Geometry check sheet. Reference: the model listing, model coordinates, mm. Coordinates: 2 decimals unless noted, no trailing zeros. Write each loop counter-clockwise with the first axis right and the second up, starting at its lowest first coordinate (ties: lowest second). Pieces come first, ordered by that corner, then holes. Notation, with made-up numbers: (-1, 64) -> (43, 64) arc R38 ccw to (43, 102) -> close; hole circle Ø7 at (-21, 10). An arc over 180 degrees is marked (long way). Use a Markdown table: item, result.
```python
from build123d import *

# Parameters (mm, degrees)
SKETCH2_R           = 1.5
SKETCH2_R_2         = 1
SKETCH2_W           = 3
SKETCH2_H           = 4.5
BOSS_EXTRUDE1_DEPTH = 3


with BuildPart() as part:
    # Sketch2 → Boss-Extrude1 (new body)
    with BuildSketch(Plane(origin=(0, 0, 0), x_dir=(1, 0, 0), z_dir=(0, 1, 0))):
        with BuildLine():
            Line((-90, 8.416796225), (-160, 8.416796225))
            Line((-160, 8.416796225), (-160, 40.416796225))
            Line((-160, 40.416796225), (-136, 40.416796225))
            Line((-136, 40.416796225), (-136, 43.416796225))
            Line((-136, 43.416796225), (-126, 43.416796225))
            Line((-126, 43.416796225), (-126, 40.416796225))
            Line((-126, 40.416796225), (-102, 40.416796225))
            Line((-102, 40.416796225), (-102, 43.416796225))
            Line((-102, 43.416796225), (-92, 43.416796225))
            Line((-92, 43.416796225), (-92, 40.416796225))
            Line((-92, 40.416796225), (-77, 40.416796225))
            Line((-77, 40.416796225), (-77, 37.316796225))
            Line((-77, 37.316796225), (-78.3, 37.316796225))
            Line((-78.3, 37.316796225), (-78.3, 34.816796225))
            Line((-78.3, 34.816796225), (-77, 34.816796225))
            Line((-77, 34.816796225), (-77, 31.016796225))
            Line((-77, 31.016796225), (-74, 31.016796225))
            Line((-74, 31.016796225), (-74, 34.816796225))
            Line((-74, 34.816796225), (-72.7, 34.816796225))
            Line((-72.7, 34.816796225), (-72.7, 37.316796225))
            Line((-72.7, 37.316796225), (-74, 37.316796225))
            Line((-74, 37.316796225), (-74, 40.416796225))
            Line((-74, 40.416796225), (-68, 40.416796225))
            Line((-68, 40.416796225), (-68, 43.416796225))
            Line((-68, 43.416796225), (-58, 43.416796225))
            Line((-58, 43.416796225), (-58, 40.416796225))
            Line((-58, 40.416796225), (0, 40.416796225))
            Line((0, 40.416796225), (0, 8.416796225))
            ThreePointArc((0, 8.416796225), (-2.44071054, 1.870259518), (-8.571428571, -1.480636961))
            ThreePointArc((-8.571428571, -1.480636961), (-19.756847872, -2.687843732), (-31, -3.090935939))
            Line((-31, -3.090935939), (-31, -20.090935939))
            Line((-31, -20.090935939), (-41, -20.090935939))
            Line((-41, -20.090935939), (-41, -2.772140939))
            ThreePointArc((-41, -2.772140939), (-65.95065205, 0.848775542), (-90, 8.416796225))
        make_face()
        with Locations(Location((-22.5, 8.416796225, 0), (0, 0, 270))):
            Circle(SKETCH2_R, mode=Mode.SUBTRACT)
        with Locations(Location((-15.5, 8.416796225, 0), (0, 0, 270))):
            Circle(SKETCH2_R_2, mode=Mode.SUBTRACT)
        with Locations(Location((-29.5, 8.416796225, 0), (0, 0, 90))):
            Circle(SKETCH2_R_2, mode=Mode.SUBTRACT)
        with Locations(Location((-9.5, 8.416796225, 0), (0, 0, 270))):
            Circle(SKETCH2_R_2, mode=Mode.SUBTRACT)
        with Locations(Location((-35.5, 8.416796225, 0), (0, 0, 90))):
            Circle(SKETCH2_R_2, mode=Mode.SUBTRACT)
        with Locations(Location((-154.5, 24.416796225, 0), (0, 0, 270))):
            Circle(SKETCH2_R, mode=Mode.SUBTRACT)
        with Locations((-154.5, 33.166796225)):
            Rectangle(SKETCH2_W, SKETCH2_H, mode=Mode.SUBTRACT)
        with Locations((-154.5, 15.666796225)):
            Rectangle(SKETCH2_W, SKETCH2_H, mode=Mode.SUBTRACT)
        Polygon((-32.5, -15.590935939), (-33.52606043, -18.410013802), (-36.345138292, -17.383953372), (-35.319077862, -14.564875509), align=None, mode=Mode.SUBTRACT)
        with BuildLine():
            ThreePointArc((-147, 27.116796225), (-145.581399645, 30.135325114), (-143.198066283, 32.468491571))
            ThreePointArc((-143.198066283, 32.468491571), (-142.855798146, 29.686729967), (-140.641525824, 27.968491571))
            ThreePointArc((-140.641525824, 27.968491571), (-143.745857333, 26.98342376), (-147, 27.116796225))
        make_face(mode=Mode.SUBTRACT)
        with BuildLine():
            ThreePointArc((-141.198066283, 33.500603039), (-139.132957266, 31.923161808), (-138.641525824, 29.371399432))
            ThreePointArc((-138.641525824, 29.371399432), (-136.955030568, 31.428045885), (-135.912116211, 33.874756027))
            ThreePointArc((-135.912116211, 33.874756027), (-138.582002565, 34.067876633), (-141.198066283, 33.500603039))
        make_face(mode=Mode.SUBTRACT)
    extrude(amount=BOSS_EXTRUDE1_DEPTH)


solid = part.part
```
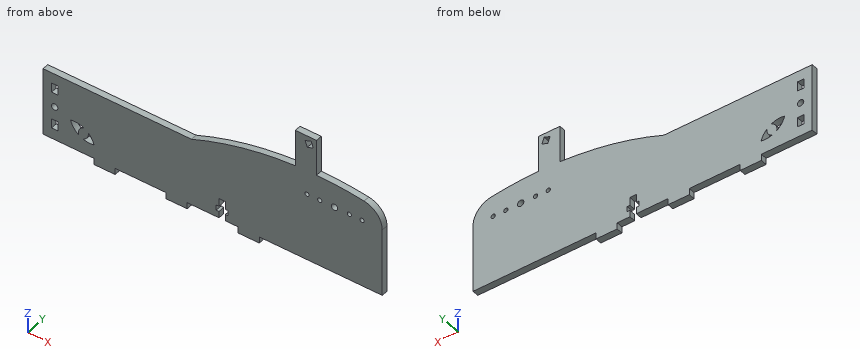
Item 1: Section check A-A on x = -22.5. Record the boundary of the cut face in (y, z), then the cut area to 3 significant figures.
Answer block:
| item | result |
|---|---|
| outline | (0, -40.42) -> (3, -40.42) -> (3, -9.92) -> (0, -9.92) -> close; (0, -6.92) -> (3, -6.92) -> (3, 2.86) -> (0, 2.86) -> close |
| area | 121 mm^2 |
Item 2: Depth check by flat-ended pin: P1, Ø3, axis at x = -85.5, z = -27, coming from the -Y side; P2, Ø1.2, axis at x = -35.5, z = -8.42, coming from the +Y side; P3, Ø0.9, axis at y = 1.5, z = -42, coming from the -X side; P4, Ø1, axis at x = -75, y = 1.5, coming from the -Z side. Enter the tip coordinate at first touch or a pass-through.
Answer block:
| item | result |
|---|---|
| P1 | stops at y = 0 |
| P2 | passes through |
| P3 | stops at x = -136 |
| P4 | stops at z = -31.02 |
Item 3: Section check C-C on y = 0.9. Count the separate pieces of the cut face and the enclosed holes in it, then the cut area to 3 significant figures.
Answer block:
| item | result |
|---|---|
| separate pieces | 1 |
| enclosed holes | 11 |
| area | 6,020 mm^2 |
Item 4: Thickness scan on L1, parallel to Z at x = -154.5, y = 1.1; L2, parallel to X at y = 1.1, z = -17; L3, parallel to Z at x = -73.5, y = 1.2. Record the ranges inside material, lowest first. Write a range as [from, to].
Answer block:
| item | result |
|---|---|
| L1 | z = [-40.42, -35.42], [-30.92, -25.92], [-22.92, -17.92], [-13.42, -8.42] |
| L2 | x = [-160, -156], [-153, 0] |
| L3 | z = [-40.42, -37.32], [-34.82, -2.77] |
Item 5: Section check B-B on x = -98. Record the boundary of the cut face in (y, z), then the cut area to 3 significant figures.
Answer block:
| item | result |
|---|---|
| outline | (0, -43.42) -> (3, -43.42) -> (3, -8.42) -> (0, -8.42) -> close |
| area | 105 mm^2 |
Item 6: Section check D-D on z = 8.5. Record the boundary of the cut face in (x, y), then the cut area to 3 significant figures.
Answer block:
| item | result |
|---|---|
| outline | (-41, 0) -> (-31, 0) -> (-31, 3) -> (-41, 3) -> close |
| area | 30.0 mm^2 |
